```python
from build123d import *

# Parameters (mm, degrees)
SKETCH1_R           = 5.5
BOSS_EXTRUDE2_DEPTH = 7
SKETCH3_W           = 3.2
SKETCH3_H           = 5.5
CUT_EXTRUDE1_DEPTH  = 6
BOSS_EXTRUDE3_DEPTH = 7


with BuildPart() as part:
    # Sketch1 → Boss-Extrude2 (new body)
    with BuildSketch(Plane.XY.offset(20)):
        with Locations((0, 20.92523633)):
            Circle(SKETCH1_R)
    extrude(amount=BOSS_EXTRUDE2_DEPTH)

    # Sketch3 → Cut-Extrude1 (cut)
    with BuildSketch(Plane.XY.offset(28.5)):
        with Locations((0, 20.92523633)):
            Rectangle(SKETCH3_W, SKETCH3_H)
    extrude(amount=-CUT_EXTRUDE1_DEPTH, mode=Mode.SUBTRACT)

    # Sketch4 → Boss-Extrude3 (add)
    with BuildSketch(Plane.XY.offset(20)):
        with BuildLine():
            Line((-0.589624168, 28.259910336), (-0.780713641, 26.369544019))
            ThreePointArc((-0.780713641, 26.369544019), (0, 26.42523633), (0.780713641, 26.369544019))
            Line((0.780713641, 26.369544019), (0.589624168, 28.259910336))
            ThreePointArc((0.589624168, 28.259910336), (0.413456372, 28.561426906), (0.106677857, 28.728262986))
            ThreePointArc((0.106677857, 28.728262986), (0, 28.731092023), (-0.106677857, 28.728262986))
            ThreePointArc((-0.106677857, 28.728262986), (-0.413456372, 28.561426906), (-0.589624168, 28.259910336))
        make_face()
        with BuildLine():
            Line((4.177966512, 26.982438264), (3.39827169, 25.249788274))
            ThreePointArc((3.39827169, 25.249788274), (2.75, 25.688376051), (2.046035999, 26.030501915))
            Line((2.046035999, 26.030501915), (3.156707495, 27.572062432))
            ThreePointArc((3.156707495, 27.572062432), (3.460031567, 27.745099543), (3.809127593, 27.736194569))
            ThreePointArc((3.809127593, 27.736194569), (3.902927847, 27.685305659), (3.993899063, 27.629516712))
            ThreePointArc((3.993899063, 27.629516712), (4.176159009, 27.331643171), (4.177966512, 26.982438264))
        make_face()
        with BuildLine():
            Line((6.646826102, 24.081943825), (5.105265585, 22.971272329))
            ThreePointArc((5.105265585, 22.971272329), (4.763139721, 23.67523633), (4.324551944, 24.32350802))
            Line((4.324551944, 24.32350802), (6.057201934, 25.103202842))
            ThreePointArc((6.057201934, 25.103202842), (6.406406841, 25.101395339), (6.704280382, 24.919135393))
            ThreePointArc((6.704280382, 24.919135393), (6.760069329, 24.828164177), (6.810958239, 24.734363924))
            ThreePointArc((6.810958239, 24.734363924), (6.819863213, 24.385267897), (6.646826102, 24.081943825))
        make_face()
        with BuildLine():
            Line((7.334674006, 20.335612162), (5.444307689, 20.14452269))
            ThreePointArc((5.444307689, 20.14452269), (5.5, 20.92523633), (5.444307689, 21.705949971))
            Line((5.444307689, 21.705949971), (7.334674006, 21.514860499))
            ThreePointArc((7.334674006, 21.514860499), (7.636190576, 21.338692702), (7.803026656, 21.031914187))
            ThreePointArc((7.803026656, 21.031914187), (7.805855693, 20.92523633), (7.803026656, 20.818558473))
            ThreePointArc((7.803026656, 20.818558473), (7.636190576, 20.511779958), (7.334674006, 20.335612162))
        make_face()
        with BuildLine():
            Line((6.057201934, 16.747269818), (4.324551944, 17.52696464))
            ThreePointArc((4.324551944, 17.52696464), (4.763139721, 18.17523633), (5.105265585, 18.879200331))
            Line((5.105265585, 18.879200331), (6.646826102, 17.768528836))
            ThreePointArc((6.646826102, 17.768528836), (6.819863213, 17.465204763), (6.810958239, 17.116108737))
            ThreePointArc((6.810958239, 17.116108737), (6.760069329, 17.022308483), (6.704280382, 16.931337267))
            ThreePointArc((6.704280382, 16.931337267), (6.406406841, 16.749077321), (6.057201934, 16.747269818))
        make_face()
        with BuildLine():
            Line((3.156707495, 14.278410228), (2.046035999, 15.819970745))
            ThreePointArc((2.046035999, 15.819970745), (2.75, 16.162096609), (3.39827169, 16.600684386))
            Line((3.39827169, 16.600684386), (4.177966512, 14.868034396))
            ThreePointArc((4.177966512, 14.868034396), (4.176159009, 14.518829489), (3.993899063, 14.220955948))
            ThreePointArc((3.993899063, 14.220955948), (3.902927847, 14.165167001), (3.809127593, 14.114278091))
            ThreePointArc((3.809127593, 14.114278091), (3.460031567, 14.105373117), (3.156707495, 14.278410228))
        make_face()
        with BuildLine():
            Line((-0.589624168, 13.590562324), (-0.780713641, 15.480928641))
            ThreePointArc((-0.780713641, 15.480928641), (0, 15.42523633), (0.780713641, 15.480928641))
            Line((0.780713641, 15.480928641), (0.589624168, 13.590562324))
            ThreePointArc((0.589624168, 13.590562324), (0.413456372, 13.289045754), (0.106677857, 13.122209674))
            ThreePointArc((0.106677857, 13.122209674), (0, 13.119380637), (-0.106677857, 13.122209674))
            ThreePointArc((-0.106677857, 13.122209674), (-0.413456372, 13.289045754), (-0.589624168, 13.590562324))
        make_face()
        with BuildLine():
            Line((-4.177966512, 14.868034396), (-3.39827169, 16.600684386))
            ThreePointArc((-3.39827169, 16.600684386), (-2.75, 16.162096609), (-2.046035999, 15.819970745))
            Line((-2.046035999, 15.819970745), (-3.156707495, 14.278410228))
            ThreePointArc((-3.156707495, 14.278410228), (-3.460031567, 14.105373117), (-3.809127593, 14.114278091))
            ThreePointArc((-3.809127593, 14.114278091), (-3.902927847, 14.165167001), (-3.993899063, 14.220955948))
            ThreePointArc((-3.993899063, 14.220955948), (-4.176159009, 14.518829489), (-4.177966512, 14.868034396))
        make_face()
        with BuildLine():
            Line((-6.646826102, 17.768528836), (-5.105265585, 18.879200331))
            ThreePointArc((-5.105265585, 18.879200331), (-4.763139721, 18.17523633), (-4.324551944, 17.52696464))
            Line((-4.324551944, 17.52696464), (-6.057201934, 16.747269818))
            ThreePointArc((-6.057201934, 16.747269818), (-6.406406841, 16.749077321), (-6.704280382, 16.931337267))
            ThreePointArc((-6.704280382, 16.931337267), (-6.760069329, 17.022308483), (-6.810958239, 17.116108737))
            ThreePointArc((-6.810958239, 17.116108737), (-6.819863213, 17.465204763), (-6.646826102, 17.768528836))
        make_face()
        with BuildLine():
            Line((-7.334674006, 21.514860499), (-5.444307689, 21.705949971))
            ThreePointArc((-5.444307689, 21.705949971), (-5.5, 20.92523633), (-5.444307689, 20.14452269))
            Line((-5.444307689, 20.14452269), (-7.334674006, 20.335612162))
            ThreePointArc((-7.334674006, 20.335612162), (-7.636190576, 20.511779958), (-7.803026656, 20.818558473))
            ThreePointArc((-7.803026656, 20.818558473), (-7.805855693, 20.92523633), (-7.803026656, 21.031914187))
            ThreePointArc((-7.803026656, 21.031914187), (-7.636190576, 21.338692702), (-7.334674006, 21.514860499))
        make_face()
        with BuildLine():
            Line((-6.057201934, 25.103202842), (-4.324551944, 24.32350802))
            ThreePointArc((-4.324551944, 24.32350802), (-4.763139721, 23.67523633), (-5.105265585, 22.971272329))
            Line((-5.105265585, 22.971272329), (-6.646826102, 24.081943825))
            ThreePointArc((-6.646826102, 24.081943825), (-6.819863213, 24.385267897), (-6.810958239, 24.734363924))
            ThreePointArc((-6.810958239, 24.734363924), (-6.760069329, 24.828164177), (-6.704280382, 24.919135393))
            ThreePointArc((-6.704280382, 24.919135393), (-6.406406841, 25.101395339), (-6.057201934, 25.103202842))
        make_face()
        with BuildLine():
            Line((-3.156707495, 27.572062432), (-2.046035999, 26.030501915))
            ThreePointArc((-2.046035999, 26.030501915), (-2.75, 25.688376051), (-3.39827169, 25.249788274))
            Line((-3.39827169, 25.249788274), (-4.177966512, 26.982438264))
            ThreePointArc((-4.177966512, 26.982438264), (-4.176159009, 27.331643171), (-3.993899063, 27.629516712))
            ThreePointArc((-3.993899063, 27.629516712), (-3.902927847, 27.685305659), (-3.809127593, 27.736194569))
            ThreePointArc((-3.809127593, 27.736194569), (-3.460031567, 27.745099543), (-3.156707495, 27.572062432))
        make_face()
    extrude(amount=BOSS_EXTRUDE3_DEPTH)


solid = part.part
```
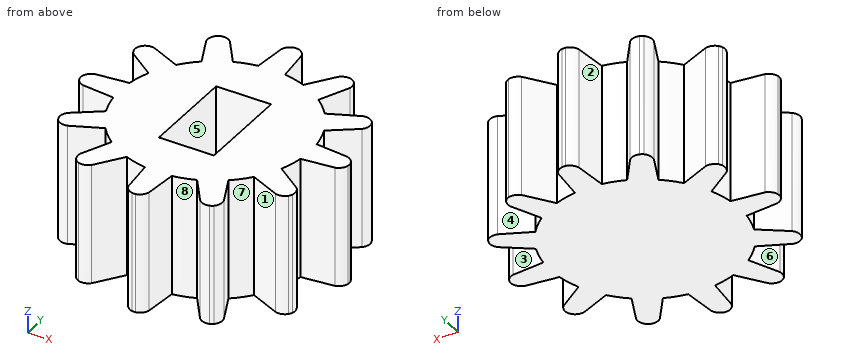
Here's how the part is built. I have some questions about the finished solid (model axes, mm). Face numbers are marked on the shaded views. A direction names the side the tool comes from. Give positions to 0.01 mm unless a question says otherwise; leave off trailing zeros. Order: outer loops, then holes, each group sorted by start corner. A loop starts at its lowest first (then second) coordinate and runs counter-clockwise, first axis right, second up. Notation, with made-up numbers: M 53.5,24 L 71.5,24 A8 ccw 71.5,33 Z; hole C 74.5,70.5 d4. An arc over 180 degrees is marked long. Use a Markdown table: item, result. Add a question column.
1. Suppose I cut it at C-C (x = -1). List the corners of the cut face in (y, z) for me, and give its area (3 significant figures).
2. Suppose I cut it at A-A (y = 15.25). List the corners of the cut face in (x, z) for me.
3. On a 3-axis mill with a long thin cutter (end or side, diameter ignored), from which of +Z, -Z, +X, -X, +Y, -Y can I reach the whole of each face in a straight line? I mean the marked faces 4, 5, 6, 7 and 8. Say none if no direction works.
4. I need wall thicknesses on probe 1 along X at (y, z) = (17, 26.25); probe 2 along Y at (x, z) = (-3.75, 22.5); probe 3 along X at (y, z) = (14.5, 23.25). Which ranges of each line are inside material? Lowest first, please. Write a range as from..to.
5. For pin 1 Ø3 at (y, z) = (16, 24.5) entering from +X; pin 2 Ø1 at (x, y) = (-0.5, 21) entering from +Z; pin 3 Ø4 at (x, z) = (5, 26) entering from +Y, each with a flat end and sliding along its axis, tell me the tip position at first contact or that it passes through.
6. If we mould it in two halves opening along Y, with no side actions, what happens to the marked faces 1, 2 and 3? For each: +Y half, -Y half, draft (parallel to the pull), parting line (faces both ways), or undercut.
7. Suppose I cut it at D-D (y = 25.75). List the corners of the cut face in (x, z) for me, and give its area (3 significant figures).
8. Suppose I cut it at B-B (y = 18.5). List the corners of the cut face in (x, z) for me, and give its area (3 significant figures).
Results list:
| question | item | result |
|---|---|---|
| 1 | outline | M 15.52,20 L 26.33,20 L 26.33,27 L 23.68,27 L 23.68,22.5 L 18.18,22.5 L 18.18,27 L 15.52,27 Z |
| 1 | area | 51.0 mm² |
| 2 | outline | M -4.01,20 L -2.46,20 L -2.46,27 L -4.01,27 Z; M -0.76,20 L 0.76,20 L 0.76,27 L -0.76,27 Z; M 2.46,20 L 4.01,20 L 4.01,27 L 2.46,27 Z |
| 3 | face 4 | +Z, -Z, +Y |
| 3 | face 5 | +Z |
| 3 | face 6 | +Z, -Z, -X |
| 3 | face 7 | +Z, -Z |
| 3 | face 8 | +Z, -Z, -Y |
| 4 | probe 1 | x = -6.75..-5.5, -3.85..3.85, 5.5..6.75 |
| 4 | probe 2 | y = 14.1..15.82, 16.9..24.95, 26.03..27.75 |
| 4 | probe 3 | x = -4.17..-3, -0.68..0.68, 3..4.17 |
| 5 | pin 1 | stops at x = 6.84 |
| 5 | pin 2 | stops at z = 22.5 |
| 5 | pin 3 | stops at y = 27.76 |
| 6 | face 1 | -Y half |
| 6 | face 2 | +Y half |
| 6 | face 3 | undercut |
| 7 | outline | M -3.62,20 L 3.62,20 L 3.62,27 L -3.62,27 Z |
| 7 | area | 50.7 mm² |
| 8 | outline | M -5.63,20 L 5.63,20 L 5.63,27 L 1.6,27 L 1.6,22.5 L -1.6,22.5 L -1.6,27 L -5.63,27 Z |
| 8 | area | 64.4 mm² |
